```python
from build123d import *

# Parameters (mm, degrees)
F1_DEPTH = 10
F2_SIZE  = 10
F3_R     = 5.5
F4_DEPTH = 7
F5_R     = 3.25
F6_DEPTH = 15
F7_R     = 2.5
F8_DEPTH = 46


with BuildPart() as f1:
    # F0 (on Front) → F1 (new body)
    with BuildSketch(Plane.XZ):
        with BuildLine():
            Line((-52.5, 25), (-52.5, -25))
            Line((-52.5, -25), (-42.5, -25))
            Line((-42.5, -25), (52.5, -25))
            Line((52.5, -25), (52.5, 4.5))
            Line((52.5, 4.5), (47.240064, 4.5))
            Line((47.240064, 4.5), (40.309475, 4.5))
            ThreePointArc((40.309475, 4.5), (26.5, 10), (40.309475, 15.5))
            Line((40.309475, 15.5), (47.240064, 15.5))
            Line((47.240064, 15.5), (52.5, 15.5))
            Line((52.5, 15.5), (52.5, 25))
            Line((52.5, 25), (-27.5, 25))
            Line((-27.5, 25), (-52.5, 25))
        make_face()
        with BuildLine():
            ThreePointArc((-39.25, -17.5), (-40.201903, -19.798097), (-42.5, -20.75))
            ThreePointArc((-42.5, -20.75), (-44.798097, -15.201903), (-39.25, -17.5))
        make_face(mode=Mode.SUBTRACT)
        with BuildLine():
            ThreePointArc((-9.25, -17.5), (-12.5, -20.75), (-15.75, -17.5))
            ThreePointArc((-15.75, -17.5), (-12.5, -14.25), (-9.25, -17.5))
        make_face(mode=Mode.SUBTRACT)
        with BuildLine():
            ThreePointArc((-25, 10), (-29.267767, 8.232233), (-27.5, 12.5))
            ThreePointArc((-27.5, 12.5), (-25.732233, 11.767767), (-25, 10))
        make_face(mode=Mode.SUBTRACT)
    extrude(amount=F1_DEPTH)

    # F2
    f2_edges = [f1.edges().sort_by_distance(p)[0] for p in [
        (-52.5, -5, 25),
    ]]
    chamfer(f2_edges, length=F2_SIZE)

    # F3 (on face) → F4 (cut)
    with BuildSketch(Plane(origin=(0, 0, 0), x_dir=(-1, 0, 0), z_dir=(0, 1, 0))):
        with Locations((12.5, -17.5)):
            Circle(F3_R)
        with Locations((42.5, -17.5)):
            Circle(F3_R)
    extrude(amount=-F4_DEPTH, mode=Mode.SUBTRACT)

    # F5 (on face) → F6 (cut)
    with BuildSketch(Plane.XY.offset(25)):
        with Locations((46.5, -5)):
            Circle(F5_R)
    extrude(amount=-F6_DEPTH, mode=Mode.SUBTRACT)

    # F7 (on face) → F8 (cut)
    with BuildSketch(Plane.XY.offset(25)):
        with Locations((46.5, -5)):
            Circle(F7_R)
    extrude(amount=-F8_DEPTH, mode=Mode.SUBTRACT)


solid = f1.part
```
Verification items for the finished model (mm, model axes). A direction names the side the tool comes from. Coordinates: 2 decimals unless noted, no trailing zeros. Write each loop counter-clockwise with the first axis right and the second up, starting at its lowest first coordinate (ties: lowest second). Pieces come first, ordered by that corner, then holes. Notation, with made-up numbers: (25.5, 66) - (65.5, 66) arc R16 cw to (65.5, 80) - close; hole circle Ø6 at (23, 19.5). An arc over 180 degrees is marked (long way). One line per question, with ' | ' between items. Start each with the question number.
1. Access from +Z, -Z, +X, -X, +Y, -Y to the whole of each face (thin tool, end or side, straight path). Record for faces 1 (the flat face through (46.3, -1.6, 15.5)), 2 (the flat face through (-45, -7, -20)), 3 (the cylindrical face through (49.502, -6.245, 20.316)).
2. Section check D-D (z = -6.5). Enter the section's corners in (x, y), plus the area to 3 significant figures.
3. Section check B-B (z = 16.5). Enter the section's corners in (x, y), plus the area to 3 significant figures.
4. Material ranges on line 1 along Z through (x, y) = (-42.5, -4.75); line 2 along Z through (x, y) = (41, -8); line 3 along Y through (x, z) = (46.5, 21.75), recorded low to high.
5. Gauge pin test, flat ends, axial feed: P1, Ø2.5, axis at x = 47.5, y = -5, coming from the +Z side; P2, Ø17.5, axis at x = -42.5, z = -17.5, coming from the +Y side; P3, Ø10, axis at x = -12.5, z = -17.5, coming from the +Y side. Record the tip position at first contact, or that the pin passes through.
6. Section check A-A (x = 46.5). Enter the section's corners in (y, z).
7. Section check C-C (x = -12.5). Enter the section's corners in (y, z), plus the area to 4 significant figures.
8. Draft check along Z on faces 4 (the cylindrical face through (-37.005, -3.451, -17.258)), 5 (the flat face through (-1, -5, -25)), 6 (the flat face through (-47.4, -4.9, 20.1)), 7 (the cylindrical face through (48.81, -5.96, -8.07)). Enter one of: released by +Z, released by -Z, zero draft, split by the parting line, or undercut.
Computed values:
1) face 1: +X, +Y, -Y | face 2: +Y | face 3: +Z
2) outline: (-52.5, -10) - (52.5, -10) - (52.5, 0) - (-52.5, 0) - close; hole circle Ø5 at (46.5, -5) | area: 1,030 mm²
3) outline: (-51, -10) - (29.84, -10) - (29.84, 0) - (-51, 0) - close; (39.16, -10) - (52.5, -10) - (52.5, 0) - (39.16, 0) - close; hole circle Ø6.5 at (46.5, -5) | area: 909 mm²
4) line 1: -25 to -23, -12 to 25 | line 2: -25 to 4.5, 15.5 to 25 | line 3: -10 to -8.25, -1.75 to 0
5) P1: z = -21 | P2: y = 0 | P3: y = -7
6) outline: (-10, -25) - (0, -25) - (0, 4.5) - (-2.5, 4.5) - (-2.5, -21) - (-7.5, -21) - (-7.5, 4.5) - (-10, 4.5) - close; (-10, 15.5) - (-8.25, 15.5) - (-8.25, 25) - (-10, 25) - close; (-1.75, 15.5) - (0, 15.5) - (0, 25) - (-1.75, 25) - close
7) outline: (-10, -25) - (0, -25) - (0, -23) - (-7, -23) - (-7, -20.75) - (-10, -20.75) - close; (-10, -14.25) - (-7, -14.25) - (-7, -12) - (0, -12) - (0, 25) - (-10, 25) - close | area: 403.5 mm²
8) face 4: undercut | face 5: released by -Z | face 6: released by +Z | face 7: zero draft
